from build123d import *

# Parameters (mm, degrees)
ESBO_O1_W                = 25
ESBO_O1_H                = 20
RESSALTO_EXTRUS_O1_DEPTH = 15
FILETE1_R                = 1
ESBO_O2_W                = 23
ESBO_O2_H                = 18
CORTE_EXTRUS_O1_DEPTH    = 10
FILETE2_R                = 1
CORTE_EXTRUS_O6_START    = -1
ESBO_O6_R                = 4
CORTE_EXTRUS_O6_DEPTH    = 3.5
ESBO_O7_W                = 23
ESBO_O7_H                = 5
CORTE_EXTRUS_O7_DEPTH    = 2


with BuildPart() as part:
    # Esboço1 → Ressalto-extrusão1 (new body)
    with BuildSketch(Plane.XY):
        Rectangle(ESBO_O1_W, ESBO_O1_H)
    extrude(amount=RESSALTO_EXTRUS_O1_DEPTH)

    # Filete1
    filete1_edges = [part.edges().sort_by_distance(p)[0] for p in [
        (-12.5, 10, 7.5),
        (12.5, 10, 7.5),
        (12.5, -10, 7.5),
        (-12.5, -10, 7.5),
    ]]
    fillet(filete1_edges, radius=FILETE1_R)

    # Esboço2 → Corte-extrusão1 (cut)
    with BuildSketch(Plane.XY.offset(15)):
        Rectangle(ESBO_O2_W, ESBO_O2_H)
    extrude(amount=-CORTE_EXTRUS_O1_DEPTH, mode=Mode.SUBTRACT)

    # Filete2
    filete2_edges = [part.edges().sort_by_distance(p)[0] for p in [
        (-11.5, -9, 10),
        (-11.5, 9, 10),
        (11.5, 9, 10),
        (11.5, -9, 10),
    ]]
    fillet(filete2_edges, radius=FILETE2_R)

    # Esboço6 → Corte-extrusão6 (cut)
    with BuildSketch(Plane.XY.offset(CORTE_EXTRUS_O6_START)):
        Circle(ESBO_O6_R)
        with Locations((7.304465977, 5.259215503)):
            Circle(ESBO_O6_R)
        with Locations((7.284465974, -5.310841468)):
            Circle(ESBO_O6_R)
    corte_extrus_o6 = extrude(amount=CORTE_EXTRUS_O6_DEPTH, mode=Mode.SUBTRACT)

    # Espelhar1: Corte-extrusão6 across plane
    add(corte_extrus_o6.mirror(Plane(origin=(0, 0, 0), x_dir=(0, 0, 1), z_dir=(1, 0, 0))), mode=Mode.SUBTRACT)

    # Esboço7 → Corte-extrusão7 (cut)
    with BuildSketch(Plane(origin=(0, 10, 0), x_dir=(1, 0, 0), z_dir=(0, 1, 0))):
        with Locations((0, -12.5)):
            Rectangle(ESBO_O7_W, ESBO_O7_H)
    extrude(amount=-CORTE_EXTRUS_O7_DEPTH, mode=Mode.SUBTRACT)


solid = part.part
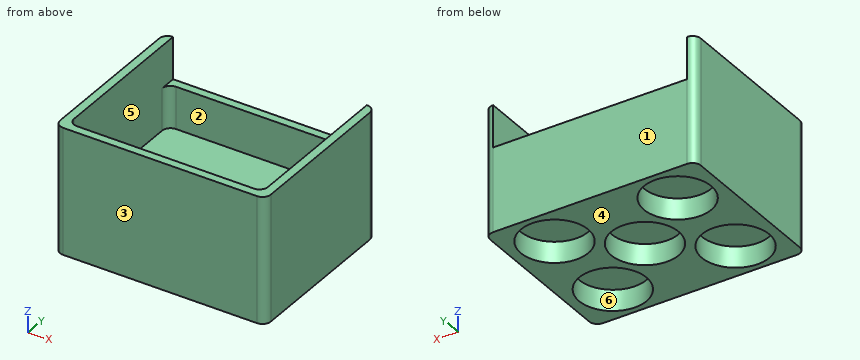
Geometry: final body of the model. Coordinates: model frame, mm. Face numbers are marked on the shaded views. A direction names the side the tool comes from. Give positions to 0.01 mm unless a question says otherwise; leave off trailing zeros. Order: outer loops, then holes, each group sorted by start corner. A loop starts at its lowest first (then second) coordinate and runs counter-clockwise, first axis right, second up. Notation, with made-up numbers: (30, 37.25) -> (40, 37.25) arc R19 ccw to (40, 61.25) -> close; hole circle Ø9 at (76.25, -24.5). An arc over 180 degrees is marked (long way). Put each result on its own line as item: value.
Q1. Draft query along Y for the marked faces 1, 2 and 3. Return one class per face: released by +Y, released by -Y, zero draft, split by the parting line, or undercut.
Here are the results:
face 1: released by +Y
face 2: undercut
face 3: released by -Y
Q2. Section D-D, the plane z = 1.5. Return loops of the section in (x, y), then the cut area to 3 significant figures.
Here are the results:
outline: (-12.5, -9) arc R1 ccw to (-11.5, -10) -> (11.5, -10) arc R1 ccw to (12.5, -9) -> (12.5, 9) arc R1 ccw to (11.5, 10) -> (-11.5, 10) arc R1 ccw to (-12.5, 9) -> close; hole circle Ø8 at (-7.3, 5.26); hole circle Ø8 at (-7.28, -5.31); hole circle Ø8 at (0, 0); hole circle Ø8 at (7.28, -5.31); hole circle Ø8 at (7.3, 5.26)
area: 248 mm^2
Q3. Pin query (flat end, axial travel): pin 1 (5 mm diameter, centred on x = 7.28, y = -5.31, fed in from +Z); pin 2 (5 mm diameter, centred on x = 7.3, y = 5.26, fed in from -Z); pin 3 (2 mm diameter, centred on x = 1.5, y = 9, fed in from +Z). Return the tip coordinate at first contact, or that it passes through.
Here are the results:
pin 1: stops at z = 5
pin 2: stops at z = 2.5
pin 3: stops at z = 10
Q4. Section C-C, the plane y = 0. Return loops of the section in (x, z).
Here are the results:
outline: (-12.5, 0) -> (-4, 0) -> (-4, 2.5) -> (4, 2.5) -> (4, 0) -> (12.5, 0) -> (12.5, 15) -> (11.5, 15) -> (11.5, 5) -> (-11.5, 5) -> (-11.5, 15) -> (-12.5, 15) -> close
Q5. Section B-B, the plane x = 0. Return loops of the section in (y, z), then the cut area to 3 significant figures.
Here are the results:
outline: (-10, 0) -> (-4, 0) -> (-4, 2.5) -> (4, 2.5) -> (4, 0) -> (10, 0) -> (10, 10) -> (9, 10) -> (9, 5) -> (-9, 5) -> (-9, 15) -> (-10, 15) -> close
area: 95.0 mm^2
Q6. Reachability of the marked faces 4, 5 and 6 from +Z, -Z, +X, -X, +Y, -Y: full face, straight path, thin tool, end or side. Return the list, or none.
Here are the results:
face 4: -Z, +X, -X, +Y, -Y
face 5: +Z
face 6: -Z
Q7. Material intervals for L1, parallel to X at y = 7.5, z = 11; L2, parallel to Y at x = 9.5, z = 6; L3, parallel to Z at x = -7.25, y = -6.25, sorted ascending.
Here are the results:
L1: x = -12.5 to -11.5, 11.5 to 12.5
L2: y = -10 to -9, 9 to 10
L3: z = 2.5 to 5
Q8. Section A-A, the plane z = 7.5. Return loops of the section in (x, y), then the cut area to 3 significant figures.
Here are the results:
outline: (-12.5, -9) arc R1 ccw to (-11.5, -10) -> (11.5, -10) arc R1 ccw to (12.5, -9) -> (12.5, 9) arc R1 ccw to (11.5, 10) -> (-11.5, 10) arc R1 ccw to (-12.5, 9) -> close; hole (-11.5, -8) arc R1 ccw to (-10.5, -9) -> (10.5, -9) arc R1 ccw to (11.5, -8) -> (11.5, 8) arc R1 ccw to (10.5, 9) -> (-10.5, 9) arc R1 ccw to (-11.5, 8) -> close
area: 86.0 mm^2
